from build123d import *

# Parameters (mm, degrees)
SKETCH1_W           = 89
SKETCH1_H           = 89
SKETCH1_W_2         = 83
SKETCH1_H_2         = 83
BOSS_EXTRUDE1_DEPTH = 22.5
SKETCH4_W           = 6
SKETCH4_H           = 6
SKETCH4_R           = 1.7
BOSS_EXTRUDE3_DEPTH = 4
FILLET3_R           = 3
SKETCH6_W           = 9
SKETCH6_H           = 17
SKETCH6_R           = 2.85
BOSS_EXTRUDE4_DEPTH = 5
CHAMFER1_SIZE       = 5
FILLET4_R           = 3
SKETCH7_R           = 1.25
CUT_EXTRUDE1_DEPTH  = 128.860275301
FILLET5_R           = 0.5


with BuildPart() as part:
    # Sketch1 → Boss-Extrude1 (new, symmetric)
    with BuildSketch(Plane(origin=(0, 0, 0), x_dir=(1, 0, 0), z_dir=(0, 1, 0))):
        with Locations((44.5, 44.5)):
            Rectangle(SKETCH1_W, SKETCH1_H)
        with Locations((44.5, 44.5)):
            Rectangle(SKETCH1_W_2, SKETCH1_H_2, mode=Mode.SUBTRACT)
    extrude(amount=BOSS_EXTRUDE1_DEPTH, both=True)

    # Sketch4 → Boss-Extrude3 (add)
    # profile 1 of 4: a face of its own
    with BuildSketch(Plane.XZ.offset(22.5)):
        with Locations((83, -6)):
            Rectangle(SKETCH4_W, SKETCH4_H)
        with Locations(Location((83, -6, 0), (0, 0, 270))):
            Circle(SKETCH4_R, mode=Mode.SUBTRACT)
    # profile 2 of 4: a face of its own
    with BuildSketch(Plane.XZ.offset(22.5)):
        with Locations((6, -6)):
            Rectangle(SKETCH4_W, SKETCH4_H)
        with Locations(Location((6, -6, 0), (0, 0, 270))):
            Circle(SKETCH4_R, mode=Mode.SUBTRACT)
    # profile 3 of 4: a face of its own
    with BuildSketch(Plane.XZ.offset(22.5)):
        with Locations((83, -83)):
            Rectangle(SKETCH4_W, SKETCH4_H)
        with Locations(Location((83, -83, 0), (0, 0, 270))):
            Circle(SKETCH4_R, mode=Mode.SUBTRACT)
    # profile 4 of 4: a face of its own
    with BuildSketch(Plane.XZ.offset(22.5)):
        with Locations((6, -83)):
            Rectangle(SKETCH4_W, SKETCH4_H)
        with Locations(Location((6, -83, 0), (0, 0, 270))):
            Circle(SKETCH4_R, mode=Mode.SUBTRACT)
    extrude(amount=-BOSS_EXTRUDE3_DEPTH)

    # Fillet3
    fillet3_edges = [part.edges().sort_by_distance(p)[0] for p in [
        (9, -20.5, -9),
        (80, -20.5, -9),
        (9, -20.5, -80),
        (80, -20.5, -80),
    ]]
    fillet(fillet3_edges, radius=FILLET3_R)

    # Sketch6 → Boss-Extrude4 (add)
    with BuildSketch(Plane.XY):
        with Locations((44.5, 14)):
            Rectangle(SKETCH6_W, SKETCH6_H)
        with Locations((44.5, 18.5)):
            Circle(SKETCH6_R, mode=Mode.SUBTRACT)
        with Locations((44.5, 9.5)):
            Circle(SKETCH6_R, mode=Mode.SUBTRACT)
    extrude(amount=BOSS_EXTRUDE4_DEPTH)

    # Chamfer1
    chamfer1_edges = [part.edges().sort_by_distance(p)[0] for p in [
        (44.5, 5.5, 0),
    ]]
    chamfer(chamfer1_edges, length=CHAMFER1_SIZE - 0.0001)  # a hair under: the kernel refuses the full size

    # Fillet4
    fillet4_edges = [part.edges().sort_by_distance(p)[0] for p in [
        (0, 0, -89),
        (89, 0, -89),
        (89, 0, 0),
        (0, 0, 0),
    ]]
    fillet(fillet4_edges, radius=FILLET4_R)

    # Sketch7 → Cut-Extrude1 (cut, through all)
    with BuildSketch(Plane(origin=(89, 0, 0), x_dir=(0, 0, -1), z_dir=(1, 0, 0))):
        with Locations((83, 19.5)):
            Circle(SKETCH7_R)
        with Locations((6, 19.5)):
            Circle(SKETCH7_R)
    extrude(amount=-CUT_EXTRUDE1_DEPTH, mode=Mode.SUBTRACT)

    # Fillet5
    fillet5_edges = [part.edges().sort_by_distance(p)[0] for p in [
        (0, 19.5, -81.75),
        (89, 19.5, -81.75),
        (0, 19.5, -4.75),
        (89, 19.5, -4.75),
    ]]
    fillet(fillet5_edges, radius=FILLET5_R)


solid = part.part
Geometry check sheet. Reference: the model listing, model coordinates, mm. A direction names the side the tool comes from. Give positions to 0.01 mm unless a question says otherwise; leave off trailing zeros. Write each loop counter-clockwise with the first axis right and the second up, starting at its lowest first coordinate (ties: lowest second). Pieces come first, ordered by that corner, then holes. Notation, with made-up numbers: (48.5, 79.25) - (105.5, 79.25) arc R13 cw to (105.5, 84.25) - close; hole circle Ø3 at (-32, -36). An arc over 180 degrees is marked (long way). Put each result on its own line as item: value.
1. Sectioned sample at B-B, the plane y = -8.5. Enter the section's corners in (x, z), plus the area to 3 significant figures.
Ans:
outline: (0, -86) arc R3 ccw to (3, -89) - (86, -89) arc R3 ccw to (89, -86) - (89, -3) arc R3 ccw to (86, 0) - (3, 0) arc R3 ccw to (0, -3) - close; hole (3, -86) - (86, -86) - (86, -3) - (3, -3) - close
area: 1,020 mm²
2. Thickness scan on line 1 (X direction, y = -21, z = -6); line 2 (X direction, y = 5.5, z = -35.5); line 3 (Z direction, x = 69.5, y = 3.5). Record the ranges inside material, lowest first.
Ans:
line 1: x = 0 to 4.3, 7.7 to 9, 80 to 81.3, 84.7 to 89
line 2: x = 0 to 3, 86 to 89
line 3: z = -89 to -86, -3 to 0
3. Set-up check for faces 1 (the cylindrical face through (87.268, 19.021, -84.155)), 2 (the flat face through (4.6, -18.5, -4.6)), 3 (the flat face through (4, -21, -9)): record each of +Z, -Z, +X, -X, +Y, -Y from which the full face is reachable in a straight line by a thin tool's end or side.
Ans:
face 1: +X, -X
face 2: +Y
face 3: +Y, -Y
4. Go/stop test with flat-tipped pins: pin 1 (5.5 mm diameter, centred on x = 83, z = -83, fed in from +Y); pin 2 (2 mm diameter, centred on y = 19.5, z = -83, fed in from +X); pin 3 (3 mm diameter, centred on x = 59.5, y = 10, fed in from +Z); pin 4 (2.5 mm diameter, centred on y = 9, z = 2.5, fed in from +X). Record where each tip stops, or that it passes through.
Ans:
pin 1: stops at y = -18.5
pin 2: passes through
pin 3: stops at z = 0
pin 4: stops at x = 49
5. Sectioned sample at D-D, the plane y = -20. Enter the section's corners in (x, z), plus the area to 3 significant figures.
Ans:
outline: (0, -86) arc R3 ccw to (3, -89) - (86, -89) arc R3 ccw to (89, -86) - (89, -3) arc R3 ccw to (86, 0) - (3, 0) arc R3 ccw to (0, -3) - close; hole (3, -80) - (6, -80) arc R3 cw to (9, -83) - (9, -86) - (80, -86) - (80, -83) arc R3 cw to (83, -80) - (86, -80) - (86, -9) - (83, -9) arc R3 cw to (80, -6) - (80, -3) - (9, -3) - (9, -6) arc R3 cw to (6, -9) - (3, -9) - close; hole circle Ø3.4 at (6, -83); hole circle Ø3.4 at (6, -6); hole circle Ø3.4 at (83, -83); hole circle Ø3.4 at (83, -6)
area: 1,120 mm²
6. Draft check along X on faces 4 (the flat face through (44, 0, 0)), 5 (the flat face through (40, 14, 2)), 6 (the flat face through (9, -21, -85)). Enter one of: +X half, -X half, draft (parallel to the pull), parting line (faces both ways), or undercut.
Ans:
face 4: draft
face 5: -X half
face 6: undercut
7. Sectioned sample at C-C, the plane z = -29. Enter the section's corners in (x, y).
Ans:
outline: (0, -22.5) - (3, -22.5) - (3, 22.5) - (0, 22.5) - close; (86, -22.5) - (89, -22.5) - (89, 22.5) - (86, 22.5) - close
